The model under review builds one solid part; all positions refer to its coordinate system, in mm. Face numbers are marked on the shaded views. A direction names the side the tool comes from. Coordinates: 2 decimals unless noted, no trailing zeros. Loops run counter-clockwise (first coordinate to the right, second up) from the corner with the lowest first, then second, coordinate; pieces in that order, holes last. Notation, with made-up numbers: M 84,-25.75 L 104,-25.75 A28 ccw 104,13.25 Z; hole C -36.75,75 d2. An arc over 180 degrees is marked long. Return JSON: item names as keys, results as strings.
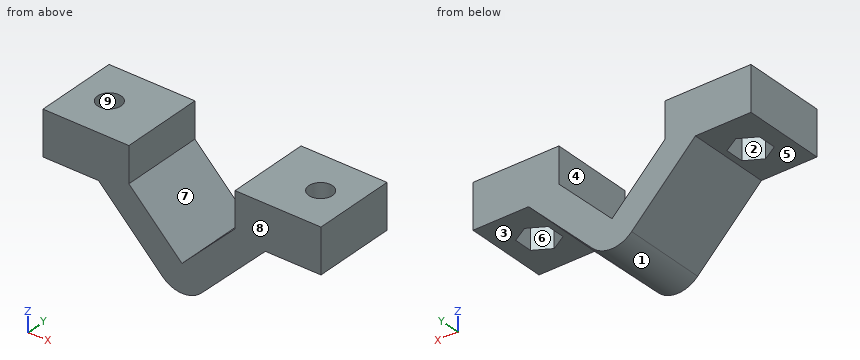
```python
from build123d import *

# Parameters (mm, degrees)
F1_DEPTH = 15
F2_R     = 2.125
F3_DEPTH = 25
F5_DEPTH = 4
F6_R     = 5
F8_DEPTH = 25


# Not quite as in the source:
# - a feature names something its author has since deleted; it is built from what else it names


with BuildPart() as f1:
    # F0 (on Front) → F1 (new body)
    with BuildSketch(Plane.XZ):
        Polygon((25, 12.8176623509), (15, 12.8176623509), (9.545941546, 12.8176623509), (9.545941546, 6.4346717088), (0, -3.1112698372), (-9.545941546, 6.4346717088), (-9.545941546, 12.8176623509), (-15, 12.8176623509), (-25, 12.8176623509), (-25, 4.8176623509), (-15, 4.8176623509), (-7.5, -2.6823376491), (0, -10.1823376491), (7.5, -2.6823376491), (15, 4.8176623509), (25, 4.8176623509), align=None)
    extrude(amount=F1_DEPTH)

    # F2 (on face) → F3 (cut)
    with BuildSketch(Plane.XY.offset(12.8176623509)):
        with Locations((-19, -7.5)):
            Circle(F2_R)
        with Locations((19, -7.5)):
            Circle(F2_R)
    extrude(amount=-F3_DEPTH, mode=Mode.SUBTRACT)

    # F4 (on face) → F5 (cut)
    with BuildSketch(Plane(origin=(0, 0, 4.8176623509), x_dir=(1, 0, 0), z_dir=(0, 0, -1))):
        Polygon((-21.925, 9.1887495374), (-21.925, 5.8112504626), (-19, 4.1225009252), (-16.075, 5.8112504626), (-16.075, 9.1887495374), (-19, 10.8774990748), align=None)
        Polygon((21.925, 5.8112504626), (21.925, 9.1887495374), (19, 10.8774990748), (16.075, 9.1887495374), (16.075, 5.8112504626), (19, 4.1225009252), align=None)
    extrude(amount=-F5_DEPTH, mode=Mode.SUBTRACT)

    # F6
    f6_edges = [f1.edges().sort_by_distance(p)[0] for p in [
        (0, -7.5, -10.182338),
    ]]
    fillet(f6_edges, radius=F6_R)

    # F7 (on face) → F8 (cut)
    with BuildSketch(Plane(origin=(0, 0, 8.8176623509), x_dir=(1, 0, 0), z_dir=(0, 0, -1))):
        Polygon((-21.925, 9.1887495374), (-21.925, 5.8112504626), (-19, 4.1225009252), (-16.075, 5.8112504626), (-16.075, 9.1887495374), (-19, 10.8774990748), align=None)
    extrude(amount=F8_DEPTH, mode=Mode.SUBTRACT)


solid = f1.part
```
1. Insertion check: pin 1 Ø6 at (y, z) = (-11.5, -2.5) entering from -X; pin 2 Ø8 at (x, y) = (-13, -11.5) entering from -Z; pin 3 Ø8 at (x, y) = (21, -5) entering from -Z. Each pin has a flat end and moves straight along its axis. Give the tip position at first contact, or say it passes through.
Check values:
{"pin 1": "x = -10.68", "pin 2": "z = -1.18", "pin 3": "z = 4.82"}
2. Machinability: for the marked faces 1, 2, 3, 4 and 5, which of the approach directions +Z, -Z, +X, -X, +Y, -Y give a long, thin tool a straight path to every point of the face, cutting with its end or side? Answer none if there is none.
Check values:
{"face 1": "-Z, +Y, -Y", "face 2": "-Z", "face 3": "-Z, +X, +Y, -Y", "face 4": "+Z, +Y, -Y", "face 5": "-Z, -X, +Y, -Y"}
3. To check wall thickness, follow line 1 (Y direction, x = 19, z = 10) (3 decimals); line 2 (X direction, y = -4.5, z = 5.5); line 3 (X direction, y = -3.25, z = 8). State the ranges of each line that lie inside material, in increasing order.
Check values:
{"line 1": "-15 to -9.625, -5.375 to 0", "line 2": "-25 to -19.65, -18.35 to -8.61, 8.61 to 18.35, 19.65 to 25", "line 3": "-25 to -9.55, 9.55 to 25"}
4. Add section C-C on y = -11.5. Give the boundary of the cut face in (x, z), plus the area to 3 significant figures.
Check values:
{"outline": "M -25,4.82 L -15,4.82 L -3.54,-6.65 A5 ccw 3.54,-6.65 L 15,4.82 L 25,4.82 L 25,12.82 L 9.55,12.82 L 9.55,6.43 L 0,-3.11 L -9.55,6.43 L -9.55,12.82 L -25,12.82 Z", "area": "407 mm²"}
5. Add section A-A on y = -7.5. State how many separate pieces and enclosed holes the cut face has, plus the area to 3 significant figures.
Check values:
{"separate pieces": "3", "enclosed holes": "0", "area": "326 mm²"}
6. Add section D-D on x = 2. Give the boundary of the cut face in (y, z).
Check values:
{"outline": "M -15,-7.69 L 0,-7.69 L 0,-1.11 L -15,-1.11 Z"}
7. The part is to be moulded in two halves that separate along Y. For the marked faces 6, 7, 8 and 9, say which applies: released by +Y, released by -Y, zero draft, split by the parting line, or undercut.
Check values:
{"face 6": "undercut", "face 7": "zero draft", "face 8": "released by -Y", "face 9": "undercut"}
8. Add section B-B on x = 20. Give the boundary of the cut face in (y, z) (3 decimals), plus the area to 3 significant figures.
Check values:
{"outline": "M -15,4.818 L -10.3,4.818 L -10.3,8.818 L -9.375,8.818 L -9.375,12.818 L -15,12.818 Z; M -5.625,8.818 L -4.7,8.818 L -4.7,4.818 L 0,4.818 L 0,12.818 L -5.625,12.818 Z", "area": "82.6 mm²"}
